For this review, take the finished solid that the model builds, in its own axes (mm). Face numbers are marked on the shaded views. A direction names the side the tool comes from. Give positions to 0.01 mm unless a question says otherwise; leave off trailing zeros. Write each loop counter-clockwise with the first axis right and the second up, starting at its lowest first coordinate (ties: lowest second). Pieces come first, ordered by that corner, then holes.
from build123d import *

# Parameters (mm, degrees)
SKETCH1_W               = 96
SKETCH1_H               = 64
BOSS_EXTRUDE1_DEPTH     = 16
CUT_EXTRUDE1_DEPTH      = 60.866518188
CUT_EXTRUDE1_DEPTH_BACK = 16
BOSS_EXTRUDE3_DEPTH     = 12
BOSS_EXTRUDE4_DEPTH     = 42
BOSS_EXTRUDE6_DEPTH     = 16


with BuildPart() as part:
    # Sketch1 → Boss-Extrude1 (new body)
    with BuildSketch(Plane(origin=(0, 0, 0), x_dir=(1, 0, 0), z_dir=(0, 1, 0))):
        Rectangle(SKETCH1_W, SKETCH1_H)
    extrude(amount=BOSS_EXTRUDE1_DEPTH)

    # Sketch2 → Cut-Extrude1 (cut, two sides: drawn at the far end of the back side and taken through both)
    with BuildSketch(Plane(origin=(0, 16, 0), x_dir=(1, 0, 0), z_dir=(0, 1, 0)).offset(-CUT_EXTRUDE1_DEPTH_BACK)):
        with BuildLine():
            Line((28, -16), (48, -16))
            Line((48, -16), (48, 0))
            Line((48, 0), (28, 0))
            ThreePointArc((28, 0), (20, -8), (28, -16))
        make_face()
    extrude(amount=CUT_EXTRUDE1_DEPTH + CUT_EXTRUDE1_DEPTH_BACK, mode=Mode.SUBTRACT)

    # Sketch3 → Boss-Extrude3 (add)
    with BuildSketch(Plane(origin=(0, 0, -32), x_dir=(-1, 0, 0), z_dir=(0, 0, -1))):
        Polygon((-48, 16), (8, 44), (8, 16), align=None)
    extrude(amount=-BOSS_EXTRUDE3_DEPTH)

    # Sketch4 → Boss-Extrude4 (add)
    with BuildSketch(Plane(origin=(0, 0, -32), x_dir=(-1, 0, 0), z_dir=(0, 0, -1))):
        with BuildLine():
            Line((8, 44), (16, 44))
            ThreePointArc((16, 44), (28, 32), (40, 44))
            Line((40, 44), (48, 44))
            Line((48, 44), (48, 16))
            Line((48, 16), (8, 16))
            Line((8, 16), (8, 44))
        make_face()
    extrude(amount=-BOSS_EXTRUDE4_DEPTH)

    # Sketch6 → Boss-Extrude6 (add)
    with BuildSketch(Plane.ZY.offset(48)):
        with BuildLine():
            Line((-32, 0), (-32, 64))
            ThreePointArc((-32, 64), (8, 50.666666667), (32, 16))
            Line((32, 16), (32, 0))
            Line((32, 0), (-32, 0))
        make_face()
    extrude(amount=BOSS_EXTRUDE6_DEPTH)


solid = part.part
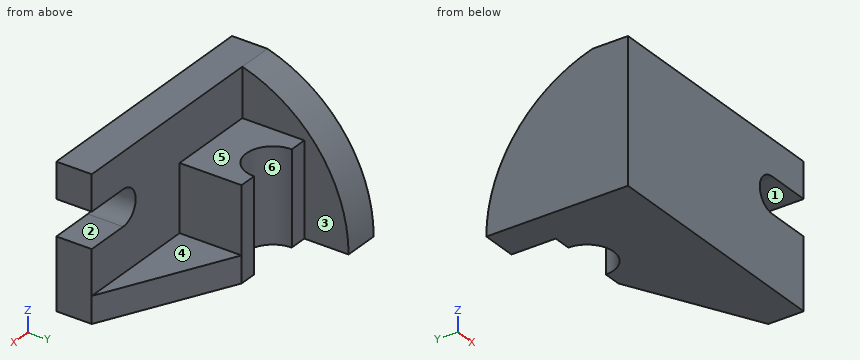
(1) We need section A-A (x = 25.5). Write out the cut boundary in (y, z), and give its area (3 significant figures).
(2) Clearance check with flat-ended pins moving along their axes: pin 1 Ø2.5 at (x, z) = (-11, -7.5) entering from +Y; pin 2 Ø3 at (x, z) = (14, 8.5) entering from +Y; pin 3 Ø14 at (x, y) = (-37, 34.5) entering from +Z. State where each tip first meets the part, or that it passes through.
(3) We need section B-B (y = 42). Write out the cut boundary in (x, z), and give its area (3 significant figures).
(4) The part is to be moulded in two halves that separate along Z. For the marked faces 1, 2, 3 and 4, say which applies: +Z half, -Z half, draft (parallel to the pull), parting line (faces both ways), or undercut.
(5) We need section D-D (x = -14.5). Write out the cut boundary in (y, z), and give its area (3 significant figures).
(6) Tool access review of the marked faces 5 and 6: name each direction out of +Z, -Z, +X, -X, +Y, -Y from which nothing blocks a thin tool from reaching the whole face with its end or side.
(7) For L1, parallel to Y at x = -28, z = -16.5; L2, parallel to Y at x = 16.5, z = 19.5; L3, parallel to X at y = 33, z = 1.5, list the stretches that pass through material, from the lowest coordinate up.
(8) We need section C-C (z = 4.5). Write out the cut boundary in (x, y).
The answers:
1. outline: (0, -32) - (27.25, -32) - (27.25, -20) - (16, -20) - (16, 0.4) - (0, 0.4) - close; (0, 15.6) - (16, 15.6) - (16, 32) - (0, 32) - close
1. area: 916 mm2
2. pin 1: stops at y = 44
2. pin 2: stops at y = 16
2. pin 3: stops at z = 10
3. outline: (-64, -32) - (-39.83, -32) - (-39.83, 10) - (-48, 10) - (-48, 17.49) - (-64, 17.49) - close; (-16.17, -32) - (-4, -32) - (-4, -20) - (-8, -20) - (-8, 10) - (-16.17, 10) - close
3. area: 1,530 mm2
4. face 1: undercut
4. face 2: undercut
4. face 3: draft
4. face 4: +Z half
5. outline: (0, -32) - (44, -32) - (44, 10) - (16, 10) - (16, 32) - (0, 32) - close
5. area: 2,200 mm2
6. face 5: +Z, +X, +Y
6. face 6: +Z, -Z, +Y
7. L1: y = 0 to 32
7. L2: y = 0 to 16
7. L3: x = -64 to -32.8, -23.2 to -8
8. outline: (-64, 0) - (20.81, 0) - (20.81, 16) - (-8, 16) - (-8, 44) - (-16, 44) arc R12 cw to (-40, 44) - (-48, 44) - (-48, 53.12) - (-64, 53.12) - close
